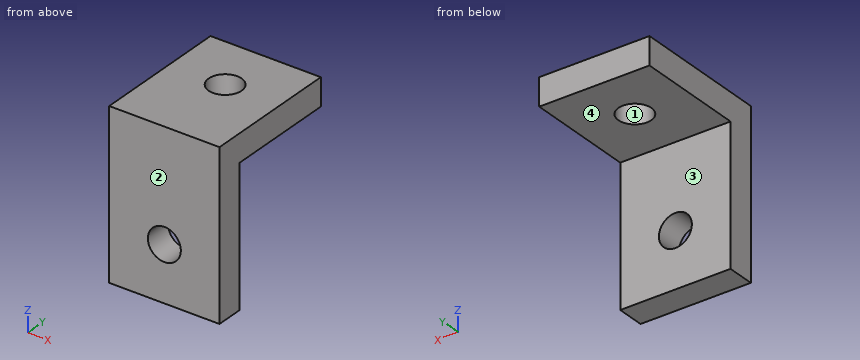
```python
from build123d import *

# Parameters (mm, degrees)
EXTRUDE1_DEPTH                      = 6.35
EXTRUDE1_DEPTH_BACK                 = 6.35
F_6_CLEARANCE_HOLE1_D               = 3.7973
F_6_CLEARANCE_HOLE1_DEPTH           = 12.7
F_6_CLEARANCE_HOLE1_TIP             = 1.140824014
F_6_CLEARANCE_HOLE1_ON_FACE_2_D     = 3.7973
F_6_CLEARANCE_HOLE1_ON_FACE_2_DEPTH = 12.7
F_6_CLEARANCE_HOLE1_ON_FACE_2_TIP   = 1.140824014


with BuildPart() as part:
    # Sketch2 → Extrude1 (new body, two sides)
    with BuildSketch(Plane(origin=(0, 0, 0), x_dir=(0, 0, -1), z_dir=(1, 0, 0))) as extrude1_sk:
        Polygon((0, 0), (0, 15.875), (3.175, 15.875), (3.175, 3.175), (19.05, 3.175), (19.05, 0), align=None)
    extrude(amount=EXTRUDE1_DEPTH)
    extrude(extrude1_sk.sketch, amount=-EXTRUDE1_DEPTH_BACK)

    # 6 Clearance Hole1
    with Locations(Plane(origin=(0, 9.525, -3.175), x_dir=(0, -1, 0), z_dir=(0, 0, -1))):
        with Locations((0, 0)):
            Hole(F_6_CLEARANCE_HOLE1_D / 2, depth=F_6_CLEARANCE_HOLE1_DEPTH)
            with Locations((0, 0, -(F_6_CLEARANCE_HOLE1_DEPTH + F_6_CLEARANCE_HOLE1_TIP / 2))):  # 118° drill point
                Cone(0, F_6_CLEARANCE_HOLE1_D / 2, F_6_CLEARANCE_HOLE1_TIP, mode=Mode.SUBTRACT)

    # 6 Clearance Hole1 on face 2
    with Locations(Plane(origin=(0, 3.175, -12.7), x_dir=(0, 0, 1), z_dir=(0, 1, 0))):
        with Locations((0, 0)):
            Hole(F_6_CLEARANCE_HOLE1_ON_FACE_2_D / 2, depth=F_6_CLEARANCE_HOLE1_ON_FACE_2_DEPTH)
            with Locations((0, 0, -(F_6_CLEARANCE_HOLE1_ON_FACE_2_DEPTH + F_6_CLEARANCE_HOLE1_ON_FACE_2_TIP / 2))):  # 118° drill point
                Cone(0, F_6_CLEARANCE_HOLE1_ON_FACE_2_D / 2, F_6_CLEARANCE_HOLE1_ON_FACE_2_TIP, mode=Mode.SUBTRACT)


solid = part.part
```
CAD build for the part. Positions are in the model's coordinates, mm. Face numbers are marked on the shaded views. Give positions to 0.01 mm unless a question says otherwise; leave off trailing zeros. Write each loop counter-clockwise with the first axis right and the second up, starting at its lowest first coordinate (ties: lowest second). Pieces come first, ordered by that corner, then holes. Notation, with made-up numbers: M -13,85.5 L 42,85.5 A17 ccw 42,113.5 Z; hole C -6,-28.75 d6. An arc over 180 degrees is marked long. Return JSON: item names as keys, results as strings. Group by question number.
(1) Band-saw the part on C-C (y = 2). Give the cut face in (x, z), and give its area (3 significant figures).
(2) Band-saw the part on A-A (z = -12.7). Give the cut face in (x, y) (3 decimals).
(3) Flat gauge pins, fed straight in: pin 1 Ø6.5 at (x, z) = (0, -14.5) entering from +Y (3 decimals); pin 2 Ø1.5 at (y, z) = (4.5, -7) entering from +X (3 decimals); pin 3 Ø1 at (x, y) = (-0.5, 8) entering from -Z (3 decimals). Where does each tip first touch, or does it go through?
(4) Band-saw the part on D-D (z = -2.5). Give the cut face in (x, y) (3 decimals).
(5) Band-saw the part on B-B (x = 0). Give the cut face in (y, z) (3 decimals), and give its area (3 significant figures).
(6) Drill centre lines: L1, parallel to X at y = 1.95, z = -12.7; L2, parallel to Z at x = 2.25, y = 12 (3 decimals); L3, parallel to Y at x = 0.75, z = -5 (3 decimals). Where is each one in solid material? Low to high. Write a range as [from, to].
(7) Mould opens along Y. For the marked faces 1, 2, 3 and 4 say: pulls with the +Y half, pulls with the -Y half, needs draft (parallel to the pull), parting line crosses it, or undercut.
Entries:
{
 "1": {"outline": "M -6.35,-19.05 L 6.35,-19.05 L 6.35,0 L -6.35,0 Z; hole C 0,-12.7 d3.8", "area": "231 mm^2"},
 "2": {"outline": "M -6.35,0 L -1.899,0 L -1.899,3.175 L -6.35,3.175 Z; M 1.899,0 L 6.35,0 L 6.35,3.175 L 1.899,3.175 Z"},
 "3": {"pin 1": "stops at y = 3.175", "pin 2": "passes through", "pin 3": "stops at z = -3.175"},
 "4": {"outline": "M -6.35,0 L 6.35,0 L 6.35,15.875 L -6.35,15.875 Z; hole C 0,9.525 d3.797"},
 "5": {"outline": "M 0,-19.05 L 3.175,-19.05 L 3.175,-14.599 L 0,-14.599 Z; M 0,-10.801 L 3.175,-10.801 L 3.175,-3.175 L 7.626,-3.175 L 7.626,0 L 0,0 Z; M 11.424,-3.175 L 15.875,-3.175 L 15.875,0 L 11.424,0 Z", "area": "76.7 mm^2"},
 "6": {"L1": "x = [-6.35, -1.9], [1.9, 6.35]", "L2": "z = [-3.175, 0]", "L3": "y = [0, 3.175]"},
 "7": {"face 1": "undercut", "face 2": "pulls with the -Y half", "face 3": "pulls with the +Y half", "face 4": "needs draft"}
}
